For this review, use the dimensioned drawing (mm, ordinates from the lowest corner) and the shaded views. Give positions to 0.01 mm unless a question says otherwise; leave off trailing zeros. Order: outer loops, then holes, each group sorted by start corner. A loop starts at its lowest first (then second) coordinate and runs counter-clockwise, first axis right, second up. Notation, with made-up numbers: (20.5, -11.75) -> (79.5, -11.75) arc R34 cw to (79.5, 21.25) -> close; hole circle Ø10 at (6.25, -13.75). An arc over 180 degrees is marked (long way). Return JSON: item names as keys, results as strings.
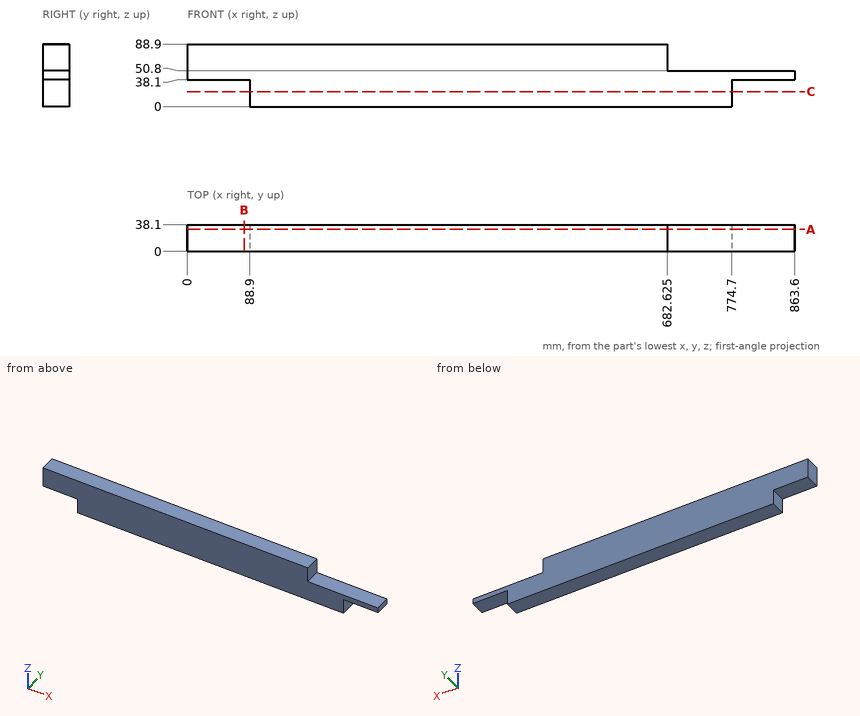
Item 1: Add section C-C (z = 21). Give the boundary of the cut face in (x, y).
Result set:
{"outline": "(88.9, 0) -> (774.7, 0) -> (774.7, 38.1) -> (88.9, 38.1) -> close"}
Item 2: Wall thickness on L1, parallel to X at y = 27.5, z = 24; L2, parallel to X at y = 31.5, z = 83 (3 decimals); L3, parallel to Z at x = 685.5, y = 2.5: over which ranges is each line inside the solid? List them lowest first. Write a range as [from, to].
Result set:
{"L1": "x = [88.9, 774.7]", "L2": "x = [0, 682.625]", "L3": "z = [0, 50.8]"}
Item 3: Add section B-B (x = 81). Give the boundary of the cut face in (y, z).
Result set:
{"outline": "(0, 38.1) -> (38.1, 38.1) -> (38.1, 88.9) -> (0, 88.9) -> close"}
Item 4: Add section A-A (y = 31). Give the boundary of the cut face in (x, z) (3 decimals), plus the area to 3 significant figures.
Result set:
{"outline": "(0, 38.1) -> (88.9, 38.1) -> (88.9, 0) -> (774.7, 0) -> (774.7, 38.1) -> (863.6, 38.1) -> (863.6, 50.8) -> (682.625, 50.8) -> (682.625, 88.9) -> (0, 88.9) -> close", "area": "63,100 mm^2"}
Item 5: For pin 1 (19 mm diameter, centred on x = 792, y = 18.5, fed in from +Z); pin 2 (5 mm diameter, centred on y = 14, z = 59, fed in from +X) (3 decimals), all flat-tipped, find the tip position at first contact; note any pin that passes through.
Result set:
{"pin 1": "stops at z = 50.8", "pin 2": "stops at x = 682.625"}
